Work out the finished part from the listing and answer in its coordinate system (mm). A direction names the side the tool comes from. Coordinates: 2 decimals unless noted, no trailing zeros. Write each loop counter-clockwise with the first axis right and the second up, starting at its lowest first coordinate (ties: lowest second). Pieces come first, ordered by that corner, then holes. Notation, with made-up numbers: (44, 4.25) - (85, 4.25) arc R22 cw to (85, 16.25) - close; hole circle Ø9 at (-5, 41). An arc over 180 degrees is marked (long way). Use one line per item in the form item = value. Start each with the question number.
Item 1: A cutting plane is placed at B-B (y = -9.5). Write down the section's boundary in (x, z), then the cut area to 3 significant figures.
Item 2: Determine the mould class of faces 1 (the cylindrical face through (53.3, -13.9, 5.7)), 2 (the cylindrical face through (-53.24, -2.735, -5.306)), 3 (the flat face through (-1, 0, -1)), 4 (the flat face through (0, -4, 54)) for opening direction Y: released by +Y, released by -Y, zero draft, split by the parting line, or undercut.
Item 3: A cutting plane is placed at C-C (z = 32). Write down the section's boundary in (x, y), then the cut area to 3 significant figures.
Item 4: Given pin 1 (2.5 mm diameter, centred on x = -32, z = 32, fed in from -Y); pin 2 (10 mm diameter, centred on x = 38, z = -6.5, fed in from -Y); pin 3 (1.6 mm diameter, centred on y = 1, z = -25.5, fed in from -X), each flat-ended and moving along its own axis, determine where each tip first touches the part or whether it passes through.
Item 5: A cutting plane is placed at A-A (x = 4.5). Write down the section's boundary in (y, z), then the cut area to 3 significant figures.
Item 6: For faces 5 (the flat face through (0, -3, 52.5)), 6 (the cylindrical face through (34.033, 0.76, 31.733)), 7 (the flat face through (-52.5, -8, 0)), determine the directions among +Z, -Z, +X, -X, +Y, -Y from which every point of the face is accessible in a straight line to the end or side of a thin tool.
Item 7: Consider probe 1 along X at (y, z) = (0.65, 32); probe 2 along X at (y, z) = (-9.75, 1); probe 3 along Y at (x, z) = (33, -21). Determine where each line is inside the solid, lowest interval first.
Item 8: A cutting plane is placed at D-D (z = 4.5). Write down the section's boundary in (x, y).
from build123d import *

# Parameters (mm, degrees)
SKETCH1_W                     = 105
SKETCH1_H                     = 105
BOSS_EXTRUDE1_DEPTH           = 1.5
SKETCH2_W                     = 20
SKETCH2_H                     = 1.5
BOSS_EXTRUDE2_DEPTH           = 8.5
SKETCH3_W                     = 1.5
SKETCH3_H                     = 20
BOSS_EXTRUDE3_DEPTH           = 17.45
SKETCH4_R                     = 1.5
CUT_EXTRUDE1_DEPTH            = 122.796561938
SKETCH5_R                     = 1.5
CUT_EXTRUDE2_DEPTH            = 122.796561938
FILLET1_R                     = 1
FILLET2_START                 = -53.84589
FILLET2_DEPTH                 = 107.69178
FILLET2_START_2               = -53
FILLET2_2_DEPTH               = 106
FILLET3_R                     = 2
SKETCH6_R                     = 2.05
HOLES_FOR_BULKHEAD_RODS_DEPTH = 10


with BuildPart() as part:
    # Sketch1 → Boss-Extrude1 (new body)
    with BuildSketch(Plane(origin=(0, 0, 0), x_dir=(1, 0, 0), z_dir=(0, 1, 0))):
        Rectangle(SKETCH1_W, SKETCH1_H)
    extrude(amount=BOSS_EXTRUDE1_DEPTH)

    # Sketch2 → Boss-Extrude2 (add)
    with BuildSketch(Plane(origin=(0, 1.5, 0), x_dir=(1, 0, 0), z_dir=(0, 1, 0))):
        with Locations((0, 53.25)):
            Rectangle(SKETCH2_W, SKETCH2_H)
        with Locations((0, -53.25)):
            Rectangle(SKETCH2_W, SKETCH2_H)
    extrude(amount=-BOSS_EXTRUDE2_DEPTH)

    # Sketch3 → Boss-Extrude3 (add)
    with BuildSketch(Plane(origin=(0, 1.5, 0), x_dir=(1, 0, 0), z_dir=(0, 1, 0))):
        with Locations((53.25, 0)):
            Rectangle(SKETCH3_W, SKETCH3_H)
        with Locations((-53.25, 0)):
            Rectangle(SKETCH3_W, SKETCH3_H)
    extrude(amount=-BOSS_EXTRUDE3_DEPTH)

    # Sketch4 → Cut-Extrude1 (cut, through all)
    with BuildSketch(Plane.XY.offset(54)):
        with Locations((-4.5, -4)):
            Circle(SKETCH4_R)
        with Locations(Location((4.5, -4, 0), (0, 0, 180))):
            Circle(SKETCH4_R)
    extrude(amount=-CUT_EXTRUDE1_DEPTH, mode=Mode.SUBTRACT)

    # Sketch5 → Cut-Extrude2 (cut, through all)
    with BuildSketch(Plane(origin=(54, 0, 0), x_dir=(0, 0, -1), z_dir=(1, 0, 0))):
        with Locations((-4.5, -4)):
            Circle(SKETCH5_R)
        with Locations((4.5, -4)):
            Circle(SKETCH5_R)
        with Locations((4.5, -13)):
            Circle(SKETCH5_R)
        with Locations((-4.5, -13)):
            Circle(SKETCH5_R)
    extrude(amount=-CUT_EXTRUDE2_DEPTH, mode=Mode.SUBTRACT)

    # Fillet1
    fillet1_edges = [part.edges().sort_by_distance(p)[0] for p in [
        (-10, -7, -53.25),
        (10, -7, -53.25),
        (-10, -7, 53.25),
        (10, -7, 53.25),
        (53.25, -15.95, -10),
        (53.25, -15.95, 10),
        (-53.25, -15.95, 10),
        (-53.25, -15.95, -10),
    ]]
    fillet(fillet1_edges, radius=FILLET1_R)

    # Fillet2: read off the stored shape, not the designer's step
    # Fillet2 outline → Fillet2 (cut)
    with BuildSketch(Plane.XY.offset(FILLET2_START)):
        with BuildLine():
            ThreePointArc((52, 1.5), (53.414213562, 0.914213562), (54, -0.5))
            Line((54, -0.5), (54, 1.5))
            Line((54, 1.5), (52, 1.5))
        make_face()
        with BuildLine():
            Line((-52, 1.5), (-54, 1.5))
            Line((-54, 1.5), (-54, -0.5))
            ThreePointArc((-54, -0.5), (-53.414213562, 0.914213562), (-52, 1.5))
        make_face()
    extrude(amount=FILLET2_DEPTH, mode=Mode.SUBTRACT)

    # Fillet2 2 outline → Fillet2 2 (cut)
    with BuildSketch(Plane.YZ.offset(FILLET2_START_2)):
        with BuildLine():
            ThreePointArc((1.5, -52), (0.914213562, -53.414213562), (-0.5, -54))
            Line((-0.5, -54), (1.5, -54))
            Line((1.5, -54), (1.5, -52))
        make_face()
        with BuildLine():
            Line((1.5, 52), (1.5, 54))
            Line((1.5, 54), (-0.5, 54))
            ThreePointArc((-0.5, 54), (0.914213562, 53.414213562), (1.5, 52))
        make_face()
    extrude(amount=FILLET2_2_DEPTH, mode=Mode.SUBTRACT)

    # Fillet3
    # the kernel refuses this fillet: 2 mm, written as the material it takes off along each edge
    with BuildSketch(Plane(origin=(52.5, -5, -52.5), x_dir=(0, 0, 1), z_dir=(0, 1, 0)), Plane(origin=(52.5, -5, 52.5), x_dir=(-1, 0, 0), z_dir=(0, 1, 0)), Plane(origin=(-52.5, -5, -52.5), x_dir=(1, 0, 0), z_dir=(0, 1, 0))) as fillet3_piece_1:
        with BuildLine():
            CenterArc((FILLET3_R, -FILLET3_R), FILLET3_R, 90, 90)
            Line((0, -FILLET3_R), (0, 0))
            Line((0, 0), (FILLET3_R, 0))
        make_face()
    extrude(amount=11.436491673, mode=Mode.SUBTRACT)
    with BuildSketch(Plane(origin=(-52.5, -5, 52.5), x_dir=(1, 0, 0), z_dir=(0, 1, 0))) as fillet3_piece_2:
        with BuildLine():
            CenterArc((FILLET3_R, FILLET3_R), FILLET3_R, 180, 90)
            Line((0, FILLET3_R), (0, 0))
            Line((0, 0), (FILLET3_R, 0))
        make_face()
    extrude(amount=11.436491673, mode=Mode.SUBTRACT)

    # Sketch6 → Holes for Bulkhead Rods (cut)
    with BuildSketch(Plane(origin=(0, 1.5, 0), x_dir=(1, 0, 0), z_dir=(0, 1, 0))):
        with Locations(Location((-32, 32, 0), (0, 0, 270))):
            Circle(SKETCH6_R)
        with Locations(Location((32, 32, 0), (0, 0, 270))):
            Circle(SKETCH6_R)
        with Locations(Location((-32, -32, 0), (0, 0, 270))):
            Circle(SKETCH6_R)
        with Locations(Location((32, -32, 0), (0, 0, 270))):
            Circle(SKETCH6_R)
    extrude(amount=-HOLES_FOR_BULKHEAD_RODS_DEPTH, mode=Mode.SUBTRACT)


solid = part.part
Answer:
q1.outline = (-54, -10) - (-52.5, -10) - (-52.5, 10) - (-54, 10) - close; (52.5, -10) - (54, -10) - (54, 10) - (52.5, 10) - close
q1.area = 60.0 mm²
q2.face_1 = undercut
q2.face_2 = undercut
q2.face_3 = released by -Y
q2.face_4 = zero draft
q3.outline = (-52.5, 0) - (-34.05, 0) - (-34.05, 1.5) - (-52, 1.5) arc R2 ccw to (-52.5, 1.44) - close; (-29.95, 0) - (29.95, 0) - (29.95, 1.5) - (-29.95, 1.5) - close; (34.05, 0) - (52.5, 0) - (52.5, 1.44) arc R2 ccw to (52, 1.5) - (34.05, 1.5) - close
q3.area = 145 mm²
q4.pin_1 = through
q4.pin_2 = 0
q4.pin_3 = -52.5
q5.outline = (-7, -54) - (-5.5, -54) - (-5.5, -52.5) - (-7, -52.5) - close; (-7, 52.5) - (-5.5, 52.5) - (-5.5, 54) - (-7, 54) - close; (-2.5, -54) - (-0.5, -54) arc R2 ccw to (1.5, -52) - (1.5, 52) arc R2 ccw to (-0.5, 54) - (-2.5, 54) - (-2.5, 52.5) - (0, 52.5) - (0, -52.5) - (-2.5, -52.5) - close
q5.area = 172 mm²
q6.face_5 = +X, -X, -Y
q6.face_6 = +Y, -Y
q6.face_7 = +Z, -Z, -Y
q7.probe_1 = -52.5 to -34.05, -29.95 to 29.95, 34.05 to 52.5
q7.probe_2 = -54 to -52.5, 52.5 to 54
q7.probe_3 = 0 to 1.5
q8.outline = (-54, -15.95) - (-52.5, -15.95) - (-52.5, -14.5) - (-54, -14.5) - close; (-54, -11.5) - (-52.5, -11.5) - (-52.5, -5.5) - (-54, -5.5) - close; (-54, -2.5) - (-52.5, -2.5) - (-52.5, 0) - (52.5, 0) - (52.5, -2.5) - (54, -2.5) - (54, -0.5) arc R2 ccw to (52, 1.5) - (-52, 1.5) arc R2 ccw to (-54, -0.5) - close; (52.5, -15.95) - (54, -15.95) - (54, -14.5) - (52.5, -14.5) - close; (52.5, -11.5) - (54, -11.5) - (54, -5.5) - (52.5, -5.5) - close
